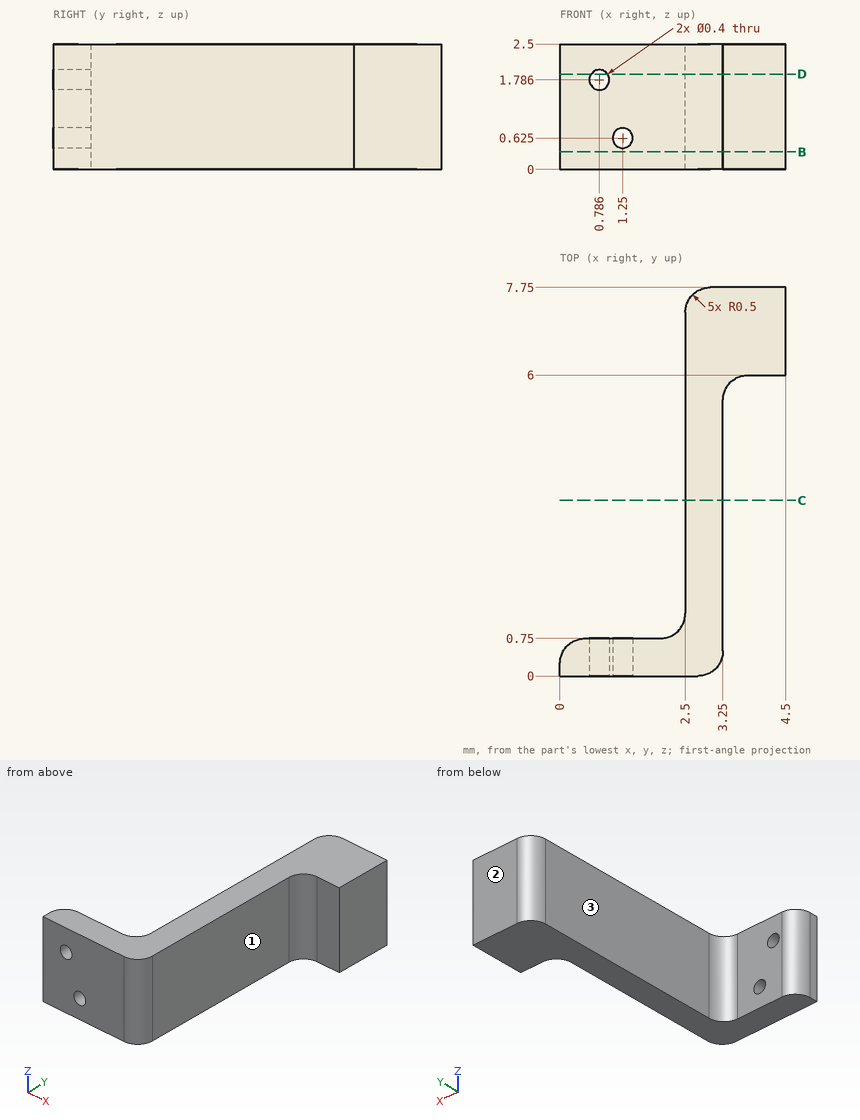
The figure shows three views and two pictorial views of one solid part (mm, origin at its lowest corner). Answer the questions. A direction names the side the tool comes from. Give positions to 0.01 mm unless a question says otherwise; leave off trailing zeros. Write each loop counter-clockwise with the first axis right and the second up, starting at its lowest first coordinate (ties: lowest second). Pieces come first, ordered by that corner, then holes.
Q1. A tool of negligible diameter and unlimited length cuts with its end or side. For the marked faces 1, 2 and 3, from which of +Z, -Z, +X, -X, +Y, -Y can it reach the whole face along a straight path? Write none if from no direction.
Answer:
face 1: +Z, -Z, +X, -Y
face 2: +Z, -Z, +X, -X, +Y
face 3: +Z, -Z, -X, +Y
Q2. The part is cut by section B-B on z = 0.35. Give the vertices of the cut face in (x, y).
Answer:
outline: (0, 0) - (2.75, 0) arc R0.5 ccw to (3.25, 0.5) - (3.25, 5.5) arc R0.5 cw to (3.75, 6) - (4.5, 6) - (4.5, 7.75) - (3, 7.75) arc R0.5 ccw to (2.5, 7.25) - (2.5, 1.25) arc R0.5 cw to (2, 0.75) - (0.5, 0.75) arc R0.5 ccw to (0, 0.25) - close
Q3. The part is cut by section C-C on y = 3.5. Give the vertices of the cut face in (x, z).
Answer:
outline: (2.5, 0) - (3.25, 0) - (3.25, 2.5) - (2.5, 2.5) - close
Q4. Straight lines are drawn through the part: L1, parallel to X at y = 3.5, z = 0.95; L2, parallel to Y at x = 3.9, z = 0.85; L3, parallel to X at y = 7, z = 0.8. For each, find the intervals that lie inside material, in ascending order.
Answer:
L1: x = 2.5 to 3.25
L2: y = 6 to 7.75
L3: x = 2.5 to 4.5
Q5. Given pin 1 (0.5 mm diameter, centred on x = 1.5, z = 0.5, fed in from +Y); pin 2 (0.8 mm diameter, centred on x = 4, z = 1.5, fed in from -Y); pin 3 (2 mm diameter, centred on x = 3.5, y = 6.5, fed in from -Z); pin 4 (0.8 mm diameter, centred on y = 4.5, z = 1, fed in from -X), each flat-ended and moving along its own axis, determine where each tip first touches the part or whether it passes through.
Answer:
pin 1: stops at y = 0.75
pin 2: stops at y = 5.98
pin 3: stops at z = 0
pin 4: stops at x = 2.5
Q6. The part is cut by section D-D on z = 1.9. Give the vertices of the cut face in (x, y).
Answer:
outline: (0, 0) - (0.62, 0) - (0.62, 0.75) - (0.5, 0.75) arc R0.5 ccw to (0, 0.25) - close; (0.95, 0) - (2.75, 0) arc R0.5 ccw to (3.25, 0.5) - (3.25, 5.5) arc R0.5 cw to (3.75, 6) - (4.5, 6) - (4.5, 7.75) - (3, 7.75) arc R0.5 ccw to (2.5, 7.25) - (2.5, 1.25) arc R0.5 cw to (2, 0.75) - (0.95, 0.75) - close
